Autodesk Inventor part; units mm, degrees
ref_plane "YZ Plane" through (0, 0, 0) normal (1, 0, 0) x (0, 1, 0)
ref_plane "XZ Plane" through (0, 0, 0) normal (0, 1, 0) x (-1, 0, 0)
ref_plane "XY Plane" through (0, 0, 0) normal (0, 0, 1) x (1, 0, 0)
sketch "Esboço1" plane through (0, 0, 0) normal (0, 0, 1) x (1, 0, 0)
  line L0 (88, 16) -> (56, 16)
  line L1 (88, -64) -> (56, -64)
  line L2 (116, -64.0154) -> (116, 11.5655)
  line L3 (-8, -88.1) -> (-8, -95.9)
  line L4 (38.5088, -95.9) -> (-8, -95.9)
  line L5 (38.5088, -95.9) -> (38.5088, -88.1)
  line L6 (38.5088, 47.9) -> (38.5088, 40.1)
  line L7 (38.5088, 47.9) -> (-8, 47.9)
  line L8 (-8, 40.1) -> (-8, 47.9)
  line L9 (99.6, 47.9) -> (99.6, 40.1)
  line L10 (-11.6, -95.9) -> (-11.6, -88.1)
  line L11 (-20, -64) -> (6.1, -90.1)
  line L12 (-20, -64) -> (16.911, -64) construction
  line L13 (-20.13, 16) -> (5.97, 42.1)
  line L14 (-20.13, 16) -> (16.781, 16) construction
  line L15 (99.3981, 42.1) -> (5.97, 42.1)
  line L16 (6.1, -90.1) -> (99.6, -90.1)
  line L17 (116, -64.0154) -> (99.6, -90.1)
  line L18 (99.3981, 42.1) -> (116, 11.5655)
  line L19 (4, -8) -> (-20.13, -8)
  line L20 (-20, -40) -> (4, -40)
  line L21 (4, -40) -> (4, -8)
  line L22 (-20.13, 16) -> (-20.13, -8)
  line L23 (-20, -40) -> (-20, -64)
  spline S0 degree 3 poles (105.3201, 14.0044) (105.3235, 14.0021) (105.3286, 13.9988) (105.3629, 13.9756) (105.3885, 13.9579) (105.4461, 13.9157) (105.482, 13.8884) (105.5584, 13.8259) (105.5988, 13.7906) (105.6725, 13.722) (105.7105, 13.6842) (105.7783, 13.6124) (105.8082, 13.5785) (105.8543, 13.5241) (105.8738, 13.4998) (105.8993, 13.4673) (105.903, 13.4624) (105.9055, 13.4591) knots -0.241565 -0.241565 -0.241565 -0.241565 -0.226467 -0.226467 -0.211369 -0.211369 -0.196271 -0.196271 -0.181173 -0.181173 -0.166076 -0.166076 -0.150978 -0.150978 -0.13588 -0.13588 -0.120782 -0.120782 -0.120782 -0.120782
  circle A0 centre (104, 12) radius 2.4
  spline S1 degree 3 poles (105.3201, -57.9956) (105.3235, -57.9979) (105.3286, -58.0012) (105.3629, -58.0244) (105.3885, -58.0421) (105.4461, -58.0843) (105.482, -58.1116) (105.5584, -58.1741) (105.5988, -58.2094) (105.6725, -58.278) (105.7105, -58.3158) (105.7783, -58.3876) (105.8082, -58.4215) (105.8543, -58.4759) (105.8738, -58.5002) (105.8993, -58.5327) (105.903, -58.5376) (105.9055, -58.5409) knots -0.241565 -0.241565 -0.241565 -0.241565 -0.226467 -0.226467 -0.211369 -0.211369 -0.196271 -0.196271 -0.181173 -0.181173 -0.166076 -0.166076 -0.150978 -0.150978 -0.13588 -0.13588 -0.120782 -0.120782 -0.120782 -0.120782
  circle A1 centre (104, -60) radius 2.4
  line L24 (64, 40.1) -> (96, 40.1)
  line L25 (-20.13, -23.115) -> (-20.13, 8)
  line L26 (56, -24) -> (88, -24)
  line L27 (115.1988, -78.8) -> (116, -78.8)
  line L28 (115.1988, 30.8) -> (116, 30.8)
  line L29 (116, 30.8) -> (105.542, 30.8)
  line L30 (116, -78.8) -> (106.7046, -78.8)
  line L31 (116, -78.8) -> (116, -64.0154)
  line L32 (116, 11.5655) -> (116, 30.8)
  point P0 (105.4155, 13.9381)
  point P1 (105.8855, 13.4849)
  point P2 (105.4436, -58.0827)
  point P3 (105.8098, -58.4238)
  dimension "d20" = 45
  dimension "d21" = 45
  dimension "d22" = 2
  dimension "d24" = 0
  dimension "d25" = 24
  dimension "d26" = 16
extrude "Extrusão1" add sketch "Esboço1" along normal blind 1.5
properties part number "PCB"
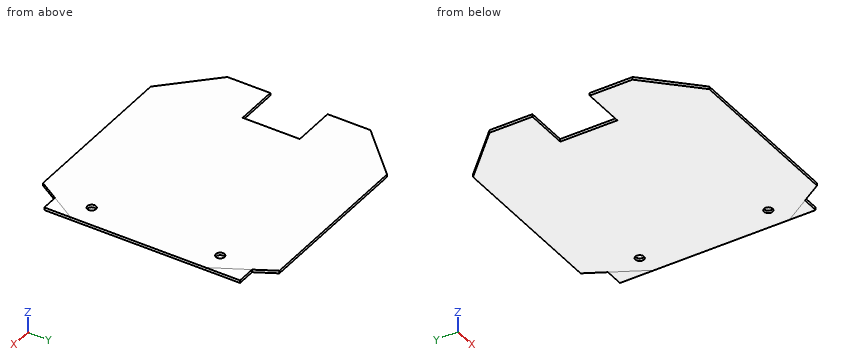
Could you check a few things on this model? Use its own coordinates, in mm. Coordinates: 2 decimals unless noted, no trailing zeros. Write each loop counter-clockwise with the first axis right and the second up, starting at its lowest first coordinate (ties: lowest second). Pieces come first, ordered by that corner, then holes. Notation, with made-up numbers: (18, 53) - (41, 53) arc R34 cw to (41, 85) - close; hole circle Ø2 at (76.25, 55.25). An arc over 180 degrees is marked (long way). Use a Markdown table: item, result.
Q1. Imagine slicing it at A-A (y = -35.5). List the corners of the cut face in (x, z) for me.
Geometry check:
| item | result |
|---|---|
| outline | (4, 0) - (116, 0) - (116, 1.5) - (4, 1.5) - close |
Q2. I'm going to push flat-ended pins straight in: pin 1 Ø0.8 at (y, z) = (-54.5, 0.5) entering from -X; pin 2 Ø12 at (x, y) = (53.5, 22) entering from -Z; pin 3 Ø0.8 at (x, z) = (109.5, 1) entering from -Y; pin 4 Ø3 at (x, y) = (104, 12) entering from -Z. Where does each tip first touch, or does it pass through?
Geometry check:
| item | result |
|---|---|
| pin 1 | stops at x = -20 |
| pin 2 | stops at z = 0 |
| pin 3 | stops at y = -78.8 |
| pin 4 | passes through |
Q3. Imagine slicing it at C-C (z = 0.3). Count the separate pieces of the cut face and the enclosed holes in it, and give its area (3 significant figures).
Geometry check:
| item | result |
|---|---|
| separate pieces | 1 |
| enclosed holes | 2 |
| area | 16,200 mm2 |
Q4. Imagine slicing it at B-B (x = 108.5). List the corners of the cut face in (y, z) for me, and give its area (3 significant figures).
Geometry check:
| item | result |
|---|---|
| outline | (-78.8, 0) - (30.8, 0) - (30.8, 1.5) - (-78.8, 1.5) - close |
| area | 164 mm2 |
Q5. Please list where these lines run through material, in increasing order: L1, parallel to Y at x = 104, z = 1.15; L2, parallel to X at y = 12, z = 0.75; L3, parallel to X at y = -37, z = 0.4.
Geometry check:
| item | result |
|---|---|
| L1 | y = -83.1 to -62.4, -57.6 to 9.6, 14.4 to 33.64 |
| L2 | x = -20.13 to 101.6, 106.4 to 116 |
| L3 | x = 4 to 116 |
